Geometry: final body of the model. Coordinates: model frame, mm. A direction names the side the tool comes from. Give positions to 0.01 mm unless a question says otherwise; leave off trailing zeros. Write each loop counter-clockwise with the first axis right and the second up, starting at its lowest first coordinate (ties: lowest second). Pieces come first, ordered by that corner, then holes.
```python
from build123d import *

# Parameters (mm, degrees)
SKETCH1_R           = 5
BOSS_EXTRUDE1_DEPTH = 210
BOSS_EXTRUDE2_DEPTH = 210
SKETCH3_R           = 3.996327594
BOSS_EXTRUDE3_DEPTH = 20


with BuildPart() as part:
    # Sketch1 → Boss-Extrude1 (new body)
    with BuildSketch(Plane.XY):
        Circle(SKETCH1_R)
    extrude(amount=-BOSS_EXTRUDE1_DEPTH)

    # Sketch2 → Boss-Extrude2 (add)
    with BuildSketch(Plane.XY):
        with BuildLine():
            Line((-5, 0), (5, 0))
            ThreePointArc((5, 0), (4.149899422, 4.734754346), (1.70579093, 8.878050545))
            ThreePointArc((1.70579093, 8.878050545), (0, 9.584612283), (-1.70579093, 8.878050545))
            ThreePointArc((-1.70579093, 8.878050545), (-4.149899422, 4.734754346), (-5, 0))
        make_face()
    extrude(amount=-BOSS_EXTRUDE2_DEPTH)

    # Sketch3 → Boss-Extrude3 (add)
    with BuildSketch(Plane.XY):
        Circle(SKETCH3_R)
    extrude(amount=BOSS_EXTRUDE3_DEPTH)


solid = part.part
```
Item 1: Reachability of faces 1 (the face through (-4.126, 4.798, -103.53)), 2 (the face through (-3.992, 0.176, 9.86)) from +Z, -Z, +X, -X, +Y, -Y: full face, straight path, thin tool, end or side. Return the list, or none.
Found:
face 1: +Z, -Z, -X, +Y
face 2: +Z
Item 2: Section A-A, the plane x = 0. Return the cut outline in (y, z), plus the area to 3 significant figures.
Found:
outline: (-5, -210) - (9.58, -210) - (9.58, 0) - (4, 0) - (4, 20) - (-4, 20) - (-4, 0) - (-5, 0) - close
area: 3,220 mm2
Item 3: Pin query (flat end, axial travel): pin 1 Ø1.5 at (x, y) = (1, 5.5) entering from +Z; pin 2 Ø1 at (y, z) = (1, -28) entering from -X; pin 3 Ø6 at (x, z) = (-4, -143) entering from +Y. Return the tip coordinate at first contact, or that it passes through.
Found:
pin 1: stops at z = 0
pin 2: stops at x = -4.99
pin 3: stops at y = 9.37
Item 4: Line query: L1, parallel to Y at x = 0.25, z = -172; L2, parallel to Z at x = -4, y = -2.25; L3, parallel to X at y = -0.25, z = -189. Output: solid intervals per line, ascending.
Found:
L1: y = -4.99 to 9.57
L2: z = -210 to 0
L3: x = -4.99 to 4.99
Item 5: Section B-B, the plane y = 2. Return the cut outline in (x, z).
Found:
outline: (-4.85, -210) - (4.85, -210) - (4.85, 0) - (3.46, 0) - (3.46, 20) - (-3.46, 20) - (-3.46, 0) - (-4.85, 0) - close
Item 6: Section C-C, the plane z = -34. Return the cut outline in (x, y), plus the area to 3 significant figures.
Found:
outline: (-5, 0) arc R5 ccw to (5, 0) arc R13.61 ccw to (1.71, 8.88) arc R2.41 ccw to (-1.71, 8.88) arc R13.61 ccw to start
area: 111 mm2
